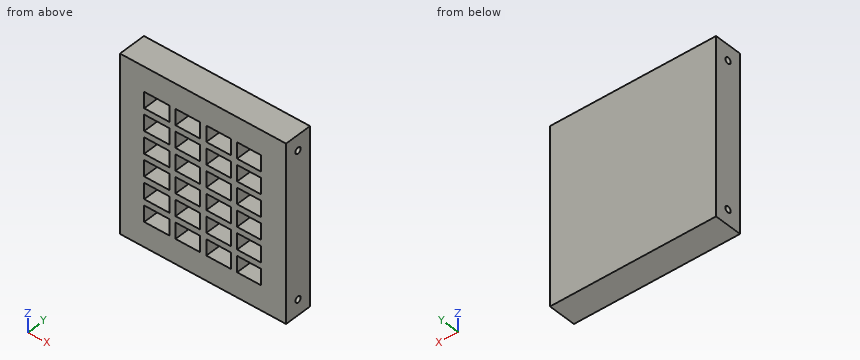
```python
from build123d import *

# Parameters (mm, degrees)
F0_W     = 171.958
F0_H     = 182.0672
F0_W_2   = 25.527
F0_H_2   = 16.5862
F1_DEPTH = 28.829
F0_W_3   = 24.7371567947
F2_DEPTH = 6.35
F3_R     = 3.175
F4_DEPTH = 203.2


# Not quite as in the source:
# - a length typed as a fraction of an inch, garbled in the dataset ("3 / 203.2 mm" for 3/8 in), is restored


with BuildPart() as f1:
    # F0 (on Front) → F1 (new body)
    with BuildSketch(Plane.XZ):
        with Locations((85.979, -91.0336)):
            Rectangle(F0_W, F0_H)
        Polygon((25.1346008565, -41.4550490677), (25.1346008565, -25.4), (51.1923991435, -25.4), (57.5423991435, -25.4), (83.0693991435, -25.4), (85.5840783974, -25.4), (89.4193991435, -25.4), (114.9463991435, -25.4), (121.2963991435, -25.4), (146.0335559382, -25.4), (146.0335559382, -41.9862), (146.0335559382, -48.1976613704), (146.0335559382, -64.9224), (146.0335559382, -71.2724), (146.0335559382, -87.8586), (146.0335559382, -94.2086), (146.0335559382, -110.7948), (146.0335559382, -117.1448), (146.0335559382, -133.731), (146.0335559382, -140.081), (146.0335559382, -156.6672), (121.2963991435, -156.6672), (114.9463991435, -156.6672), (89.4193991435, -156.6672), (83.0693991435, -156.6672), (57.5423991435, -156.6672), (51.1923991435, -156.6672), (25.1346008565, -156.6672), (25.1346008565, -140.081), (25.1346008565, -133.731), (25.1346008565, -117.1448), (25.1346008565, -110.7948), (25.1346008565, -94.2086), (25.1346008565, -87.8586), (25.1346008565, -71.2724), (25.1346008565, -64.9224), (25.1346008565, -48.3362), (25.1346008565, -41.9862), align=None, mode=Mode.SUBTRACT)
        Polygon((57.5423991435, -25.4), (51.1923991435, -25.4), (51.1923991435, -41.9862), (25.1346008565, -41.9862), (25.1346008565, -48.3362), (38.1635, -48.3362), (51.1923991435, -48.3362), (51.1923991435, -64.9224), (38.1635, -64.9224), (25.1346008565, -64.9224), (25.1346008565, -71.2724), (38.1635, -71.2724), (51.1923991435, -71.2724), (51.1923991435, -87.8586), (38.1635, -87.8586), (25.1346008565, -87.8586), (25.1346008565, -94.2086), (38.1635, -94.2086), (51.1923991435, -94.2086), (51.1923991435, -110.7948), (25.1346008565, -110.7948), (25.1346008565, -117.1448), (38.1635, -117.1448), (51.1923991435, -117.1448), (51.1923991435, -133.731), (38.1635, -133.731), (25.1346008565, -133.731), (25.1346008565, -140.081), (38.1635, -140.081), (51.1923991435, -140.081), (51.1923991435, -156.6672), (57.5423991435, -156.6672), (57.5423991435, -140.081), (83.0693991435, -140.081), (83.0693991435, -156.6672), (89.4193991435, -156.6672), (89.4193991435, -140.081), (114.9463991435, -140.081), (114.9463991435, -156.6672), (121.2963991435, -156.6672), (121.2963991435, -140.081), (146.0335559382, -140.081), (146.0335559382, -133.731), (121.2963991435, -133.731), (121.2963991435, -117.1448), (146.0335559382, -117.1448), (146.0335559382, -110.7948), (121.2963991435, -110.7948), (121.2963991435, -94.2086), (146.0335559382, -94.2086), (146.0335559382, -87.8586), (121.2963991435, -87.8586), (121.2963991435, -71.2724), (146.0335559382, -71.2724), (146.0335559382, -64.9224), (121.2963991435, -64.9224), (121.2963991435, -48.3362), (146.0335559382, -48.1976613704), (146.0335559382, -41.9862), (121.2963991435, -41.9862), (121.2963991435, -25.4), (114.9463991435, -25.4), (114.9463991435, -41.9862), (89.4193991435, -41.9862), (89.4193991435, -25.4), (85.5840783974, -25.4), (83.0693991435, -25.4), (83.0693991435, -41.9862), (57.5423991435, -41.9862), align=None)
        with Locations((70.3058991435, -125.4379)):
            Rectangle(F0_W_2, F0_H_2, mode=Mode.SUBTRACT)
        with Locations((70.3058991435, -102.5017)):
            Rectangle(F0_W_2, F0_H_2, mode=Mode.SUBTRACT)
        with Locations((102.1828991435, -125.4379)):
            Rectangle(F0_W_2, F0_H_2, mode=Mode.SUBTRACT)
        with Locations((102.1828991435, -102.5017)):
            Rectangle(F0_W_2, F0_H_2, mode=Mode.SUBTRACT)
        with Locations((70.3058991435, -79.5655)):
            Rectangle(F0_W_2, F0_H_2, mode=Mode.SUBTRACT)
        with Locations((70.3058991435, -56.6293)):
            Rectangle(F0_W_2, F0_H_2, mode=Mode.SUBTRACT)
        with Locations((102.1828991435, -79.5655)):
            Rectangle(F0_W_2, F0_H_2, mode=Mode.SUBTRACT)
        with Locations((102.1828991435, -56.6293)):
            Rectangle(F0_W_2, F0_H_2, mode=Mode.SUBTRACT)
    extrude(amount=F1_DEPTH)

    # F0 (on Front) → F2 (join)
    with BuildSketch(Plane.XZ):
        Polygon((51.1923991435, -25.4), (25.1346008565, -25.4), (25.1346008565, -41.4550490677), (25.1346008565, -41.9862), (51.1923991435, -41.9862), align=None)
        with Locations((70.3058991435, -33.6931)):
            Rectangle(F0_W_2, F0_H_2)
        with Locations((102.1828991435, -33.6931)):
            Rectangle(F0_W_2, F0_H_2)
        with Locations((133.6649775409, -33.6931)):
            Rectangle(F0_W_3, F0_H_2)
        Polygon((146.0335559382, -64.9224), (146.0335559382, -48.1976613704), (121.2963991435, -48.3362), (121.2963991435, -64.9224), align=None)
        with Locations((102.1828991435, -56.6293)):
            Rectangle(F0_W_2, F0_H_2)
        with Locations((70.3058991435, -56.6293)):
            Rectangle(F0_W_2, F0_H_2)
        Polygon((38.1635, -48.3362), (25.1346008565, -48.3362), (25.1346008565, -64.9224), (38.1635, -64.9224), (51.1923991435, -64.9224), (51.1923991435, -48.3362), align=None)
        Polygon((38.1635, -71.2724), (25.1346008565, -71.2724), (25.1346008565, -87.8586), (38.1635, -87.8586), (51.1923991435, -87.8586), (51.1923991435, -71.2724), align=None)
        with Locations((70.3058991435, -79.5655)):
            Rectangle(F0_W_2, F0_H_2)
        with Locations((102.1828991435, -79.5655)):
            Rectangle(F0_W_2, F0_H_2)
        with Locations((133.6649775409, -79.5655)):
            Rectangle(F0_W_3, F0_H_2)
        with Locations((133.6649775409, -102.5017)):
            Rectangle(F0_W_3, F0_H_2)
        with Locations((102.1828991435, -102.5017)):
            Rectangle(F0_W_2, F0_H_2)
        with Locations((70.3058991435, -102.5017)):
            Rectangle(F0_W_2, F0_H_2)
        Polygon((38.1635, -94.2086), (25.1346008565, -94.2086), (25.1346008565, -110.7948), (51.1923991435, -110.7948), (51.1923991435, -94.2086), align=None)
        Polygon((38.1635, -117.1448), (25.1346008565, -117.1448), (25.1346008565, -133.731), (38.1635, -133.731), (51.1923991435, -133.731), (51.1923991435, -117.1448), align=None)
        with Locations((133.6649775409, -125.4379)):
            Rectangle(F0_W_3, F0_H_2)
        with Locations((133.6649775409, -148.3741)):
            Rectangle(F0_W_3, F0_H_2)
        with Locations((102.1828991435, -148.3741)):
            Rectangle(F0_W_2, F0_H_2)
        with Locations((70.3058991435, -148.3741)):
            Rectangle(F0_W_2, F0_H_2)
        Polygon((38.1635, -140.081), (25.1346008565, -140.081), (25.1346008565, -156.6672), (51.1923991435, -156.6672), (51.1923991435, -140.081), align=None)
        with Locations((102.1828991435, -125.4379)):
            Rectangle(F0_W_2, F0_H_2)
        with Locations((70.3058991435, -125.4379)):
            Rectangle(F0_W_2, F0_H_2)
    extrude(amount=F2_DEPTH)

    # F3 (on face) → F4 (cut)
    with BuildSketch(Plane(origin=(0, 0, 0), x_dir=(0, -1, 0), z_dir=(-1, 0, 0))):
        with Locations((14.4145, -15.875)):
            Circle(F3_R)
        with Locations((14.4145, -166.1922)):
            Circle(F3_R)
    extrude(amount=-F4_DEPTH, mode=Mode.SUBTRACT)


solid = f1.part
```
Source: CAD feature listing. Evaluate the final solid. Frame: model axes, mm. Coordinates: 2 decimals unless noted, no trailing zeros. Order: outer loops, then holes, each group sorted by start corner. A loop starts at its lowest first (then second) coordinate and runs counter-clockwise, first axis right, second up. Notation, with made-up numbers: (25.25, 83) - (50.25, 83) arc R16 ccw to (50.25, 110) - close; hole circle Ø7 at (19, -36.75). An arc over 180 degrees is marked (long way). One line per item, written item: value.
1) Ray query, line 1 (X direction, y = -24, z = -40); line 2 (Z direction, x = 9.5, y = -12.75); line 3 (Y direction, x = 35, z = -38). Return the intervals inside material, ascending. Write a range as [from, to].
Computed values:
line 1: x = [0, 25.13], [51.19, 57.54], [83.07, 89.42], [114.95, 121.3], [146.03, 171.96]
line 2: z = [-182.07, -168.9], [-163.49, -18.58], [-13.17, 0]
line 3: y = [-6.35, 0]
2) Cut plane A-A on x = 91.5. State how many separate pieces and enclosed holes the cut face has, plus the area to 3 significant figures.
Computed values:
separate pieces: 1
enclosed holes: 2
area: 2,950 mm^2
3) Cut plane B-B on z = -29.5. Output: boundary loops of the cut face in (x, y), plus the area to 3 significant figures.
Computed values:
outline: (0, -28.83) - (25.13, -28.83) - (25.13, -6.35) - (51.19, -6.35) - (51.19, -28.83) - (57.54, -28.83) - (57.54, -6.35) - (83.07, -6.35) - (83.07, -28.83) - (89.42, -28.83) - (89.42, -6.35) - (114.95, -6.35) - (114.95, -28.83) - (121.3, -28.83) - (121.3, -6.35) - (146.03, -6.35) - (146.03, -28.83) - (171.96, -28.83) - (171.96, 0) - (0, 0) - close
area: 2,670 mm^2
4) Contact query for flat-ended pins moving along their axis: pin 1 (4 mm diameter, centred on x = 138.5, z = -77.5, fed in from +Y); pin 2 (5 mm diameter, centred on x = 65.5, z = -102, fed in from -Y). Output: stop coordinate, or through.
Computed values:
pin 1: stops at y = 0
pin 2: stops at y = -6.35
